```python
from build123d import *

# Parameters (mm, degrees)
EXTRUDE_1_DEPTH     = 40
SKETCH_2_R          = 2.6
CUT_EXTRUDE_1_DEPTH = 10
CHAMFER_1_SIZE      = 1


with BuildPart() as part:
    # 草图1 → 凸台-拉伸1 (new body, symmetric)
    with BuildSketch(Plane.XY):
        with BuildLine():
            Line((35, 0), (14.5, 0))
            ThreePointArc((14.5, 0), (0, -14.5), (-14.5, 0))
            Line((-14.5, 0), (-35, 0))
            Line((-35, 0), (-35, -5))
            Line((-35, -5), (-21.937410968, -5))
            Line((-21.937410968, -5), (-17.811513131, -5))
            ThreePointArc((-17.811513131, -5), (0, -18.5), (17.811513131, -5))
            Line((17.811513131, -5), (21.937410968, -5))
            Line((21.937410968, -5), (35, -5))
            Line((35, -5), (35, 0))
        make_face()
    extrude(amount=EXTRUDE_1_DEPTH, both=True)

    # 草图2 → 切除-拉伸1 (cut)
    with BuildSketch(Plane(origin=(0, -5, 0), x_dir=(-1, 0, 0), z_dir=(0, -1, 0))):
        with Locations((27.5, -20)):
            Circle(SKETCH_2_R)
        with Locations((27.5, 20)):
            Circle(SKETCH_2_R)
        with Locations((-27.5, -20)):
            Circle(SKETCH_2_R)
        with Locations((-27.5, 20)):
            Circle(SKETCH_2_R)
    extrude(amount=-CUT_EXTRUDE_1_DEPTH, mode=Mode.SUBTRACT)

    # 倒角1
    chamfer_1_edges = [part.edges().sort_by_distance(p)[0] for p in [
        (-35, -2.5, -40),
        (35, -2.5, -40),
        (-35, -2.5, 40),
        (35, -2.5, 40),
    ]]
    chamfer(chamfer_1_edges, length=CHAMFER_1_SIZE)


solid = part.part
```
Geometry check sheet. Reference: the model listing, model coordinates, mm. A direction names the side the tool comes from. Give positions to 0.01 mm unless a question says otherwise; leave off trailing zeros. Order: outer loops, then holes, each group sorted by start corner. A loop starts at its lowest first (then second) coordinate and runs counter-clockwise, first axis right, second up. Notation, with made-up numbers: (-6, -24) - (31, -24) arc R27 cw to (31, 5) - close; hole circle Ø3 at (-37, 30.5). An arc over 180 degrees is marked (long way). Answer in a Markdown table with one row per item. Add a question column.
Q1. Cross-section at D-D, the plane y = -13.25. Enter the section's corners in (x, z), then the cut area to 3 significant figures.
Q2. Cross-section at C-C, the plane x = -27.5. Enter the section's corners in (y, z).
Q3. Tool access check on faces 4 (the cylindrical face through (-27.162, -2.535, -22.578)), 5 (the flat face through (-27, -5, 1)), 6 (the flat face through (26, -5, 1)). Record the directions out of +Z, -Z, +X, -X, +Y, -Y that give a thin tool (end or side, any length) a straight path to the whole face; none if there is none.
Q4. Cross-section at A-A, the plane z = -20. Enter the section's corners in (x, y).
Q5. Mould release check, pull along Z, two halves, no side actions. Record for faces 1 (the flat face through (2, -15, 40)), 2 (the cylindrical face through (29.416, -2.535, 18.243)), 3 (the flat face through (-35, -2, 1)): pulls with the +Z half, pulls with the -Z half, needs draft (parallel to the pull), parting line crosses it, or undercut.
Q6. Material ranges on probe 1 along Z at (x, y) = (-27.5, -1.6); probe 2 along X at (y, z) = (-2.2, -20); probe 3 along X at (y, z) = (-3.2, -20), recorded low to high. Write a range as from..to.
Q7. Gauge pin test, flat ends, axial feed: pin 1 (1 mm diameter, centred on y = -15.5, z = -13, fed in from -X); pin 2 (6 mm diameter, centred on y = -9.5, z = -1.5, fed in from -X); pin 3 (3 mm diameter, centred on y = -8.5, z = 24.5, fed in from -X). Record the tip position at first contact, or that the pin passes through.
Q8. Cross-section at B-B, the plane y = -2.5. Enter the section's corners in (x, z).
Check values:
| question | item | result |
|---|---|---|
| 1 | outline | (-12.91, -40) - (-5.89, -40) - (-5.89, 40) - (-12.91, 40) - close; (5.89, -40) - (12.91, -40) - (12.91, 40) - (5.89, 40) - close |
| 1 | area | 1,120 mm^2 |
| 2 | outline | (-5, -40) - (0, -40) - (0, -22.6) - (-5, -22.6) - close; (-5, -17.4) - (0, -17.4) - (0, 17.4) - (-5, 17.4) - close; (-5, 22.6) - (0, 22.6) - (0, 40) - (-5, 40) - close |
| 3 | face 4 | +Y, -Y |
| 3 | face 5 | +Z, -Z, -X, -Y |
| 3 | face 6 | +Z, -Z, +X, -Y |
| 4 | outline | (-35, -5) - (-30.1, -5) - (-30.1, 0) - (-35, 0) - close; (-24.9, -5) - (-17.81, -5) arc R18.5 ccw to (17.81, -5) - (24.9, -5) - (24.9, 0) - (14.5, 0) arc R14.5 cw to (-14.5, 0) - (-24.9, 0) - close; (30.1, -5) - (35, -5) - (35, 0) - (30.1, 0) - close |
| 5 | face 1 | pulls with the +Z half |
| 5 | face 2 | undercut |
| 5 | face 3 | needs draft |
| 6 | probe 1 | z = -40..-22.6, -17.4..17.4, 22.6..40 |
| 6 | probe 2 | x = -35..-30.1, -24.9..-14.33, 14.33..24.9, 30.1..35 |
| 6 | probe 3 | x = -35..-30.1, -24.9..-14.14, 14.14..24.9, 30.1..35 |
| 7 | pin 1 | stops at x = -10.83 |
| 7 | pin 2 | stops at x = -17.32 |
| 7 | pin 3 | stops at x = -17.12 |
| 8 | outline | (-35, -39) - (-34, -40) - (-14.28, -40) - (-14.28, 40) - (-34, 40) - (-35, 39) - close; (14.28, -40) - (34, -40) - (35, -39) - (35, 39) - (34, 40) - (14.28, 40) - close; hole circle Ø5.2 at (-27.5, -20); hole circle Ø5.2 at (-27.5, 20); hole circle Ø5.2 at (27.5, -20); hole circle Ø5.2 at (27.5, 20) |
